Check sheet for the drawn part. Datum: minimum x, y, z corner. Units: mm. Round coordinates to 2 decimals unless told otherwise and drop trailing zeros. Loops run counter-clockwise (first coordinate to the right, second up) from the corner with the lowest first, then second, coordinate; pieces in that order, holes last.
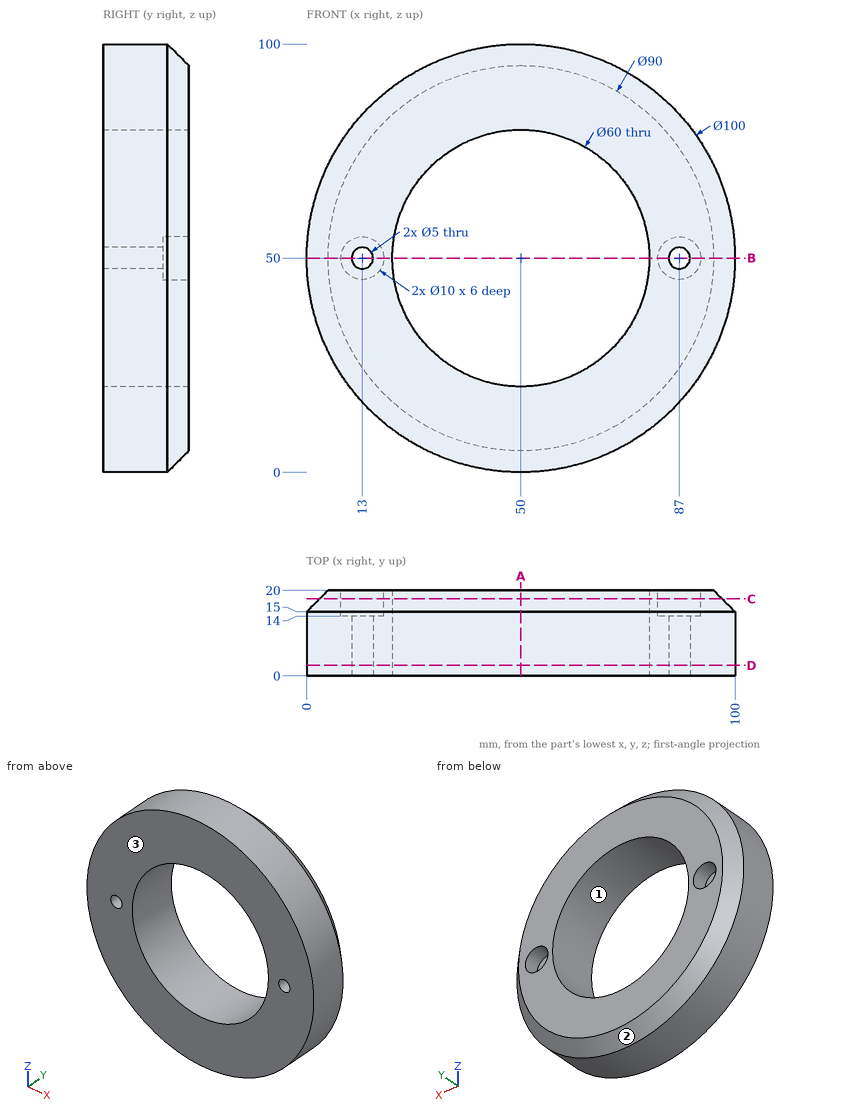
1) Sectioned sample at A-A, the plane x = 50. Record the cut outline in (y, z).
Report:
outline: (0, 0) - (15, 0) - (20, 5) - (20, 20) - (0, 20) - close; (0, 80) - (20, 80) - (20, 95) - (15, 100) - (0, 100) - close
2) Gauge pin test, flat ends, axial feed: pin 1 (4 mm diameter, centred on y = 5, z = 72.5, fed in from +X); pin 2 (12 mm diameter, centred on x = 15.5, y = 2, fed in from -Z); pin 3 (8 mm diameter, centred on y = 16.5, z = 59.5, fed in from -X); pin 4 (4.5 mm diameter, centred on x = 87, z = 50, fed in from -Y). Record the tip position at first contact, or that the pin passes through.
Report:
pin 1: stops at x = 95.6
pin 2: stops at z = 8.92
pin 3: stops at x = 0.34
pin 4: passes through
3) Sectioned sample at C-C, the plane y = 18. Record the cut outline in (x, z).
Report:
outline: circle Ø94 at (50, 50); hole circle Ø10 at (13, 50); hole circle Ø60 at (50, 50); hole circle Ø10 at (87, 50)
4) Sectioned sample at D-D, the plane y = 2.5. Record the cut outline in (x, z), then the cut area to 3 significant figures.
Report:
outline: circle Ø100 at (50, 50); hole circle Ø5 at (13, 50); hole circle Ø60 at (50, 50); hole circle Ø5 at (87, 50)
area: 4,990 mm2
5) Sectioned sample at B-B, the plane z = 50. Record the cut outline in (x, y).
Report:
outline: (0, 0) - (10.5, 0) - (10.5, 14) - (8, 14) - (8, 20) - (5, 20) - (0, 15) - close; (15.5, 0) - (20, 0) - (20, 20) - (18, 20) - (18, 14) - (15.5, 14) - close; (80, 0) - (84.5, 0) - (84.5, 14) - (82, 14) - (82, 20) - (80, 20) - close; (89.5, 0) - (100, 0) - (100, 15) - (95, 20) - (92, 20) - (92, 14) - (89.5, 14) - close
6) Scan lines: line 1 along X through (y, z) = (7, 50); line 2 along X through (y, z) = (15.75, 52); line 3 along Z through (x, y) = (25, 6.75). Record each from-to range of solid material in increasing order.
Report:
line 1: x = 0 to 10.5, 15.5 to 20, 80 to 84.5, 89.5 to 100
line 2: x = 0.79 to 8.42, 17.58 to 20.07, 79.93 to 82.42, 91.58 to 99.21
line 3: z = 6.7 to 33.42, 66.58 to 93.3
7) Mould release check, pull along Z, two halves, no side actions. Record for the marked faces 1, 2 and 3: +Z half, -Z half, draft (parallel to the pull), parting line (faces both ways), or undercut.
Report:
face 1: undercut
face 2: parting line
face 3: draft
